Part model, mm, in its own coordinate system. A direction names the side the tool comes from. Coordinates: 2 decimals unless noted, no trailing zeros. Write each loop counter-clockwise with the first axis right and the second up, starting at its lowest first coordinate (ties: lowest second). Pieces come first, ordered by that corner, then holes. Notation, with made-up numbers: (-39.5, -27) - (14.5, -27) arc R33 cw to (14.5, 10) - close; hole circle Ø1 at (0, 43.25). An arc over 180 degrees is marked (long way). Write each question's results on one line, items separated by ' | '.
from build123d import *

# Parameters (mm, degrees)
SKETCH1_R           = 67.8
BOSS_EXTRUDE1_DEPTH = 20
SKETCH1_3_R         = 67.8
SKETCH1_3_R_2       = 50
BOSS_EXTRUDE2_DEPTH = 10


with BuildPart() as part:
    # Sketch1 → Boss-Extrude1 (new body)
    with BuildSketch(Plane(origin=(0, 0, 0), x_dir=(1, 0, 0), z_dir=(0, 1, 0))):
        with BuildLine():
            Line((242.754590009, 10), (260.147485469, 10))
            ThreePointArc((260.147485469, 10), (233.604843606, 39.180755583), (194.644031062, 33.009579084))
            ThreePointArc((194.644031062, 33.009579084), (161.546937037, 24.693656308), (132.733534149, 42.979170204))
            ThreePointArc((132.733534149, 42.979170204), (79.728157262, 75.530448258), (20.130518149, 57.718174568))
            ThreePointArc((20.130518149, 57.718174568), (-21.958648504, 36.745511037), (-68.95457192, 38.398915813))
            ThreePointArc((-68.95457192, 38.398915813), (-99.933181208, 34.770010311), (-118.888121928, 10))
            Line((-118.888121928, 10), (-103.07116694, 10))
            ThreePointArc((-103.07116694, 10), (-55.158288466, 0), (-103.07116694, -10))
            Line((-103.07116694, -10), (-118.888121928, -10))
            ThreePointArc((-118.888121928, -10), (-98.946037038, -35.313177478), (-66.810190141, -37.707138198))
            ThreePointArc((-66.810190141, -37.707138198), (-22.089611981, -34.732295435), (17.640354454, -55.476199781))
            ThreePointArc((17.640354454, -55.476199781), (75.663213782, -75.951962021), (129.887825017, -46.872749853))
            ThreePointArc((129.887825017, -46.872749853), (161.497288251, -27.924259237), (197.646050954, -35.098547889))
            ThreePointArc((197.646050954, -35.098547889), (235.316798867, -38.536697893), (260.147485469, -10))
            Line((260.147485469, -10), (242.754590009, -10))
            ThreePointArc((242.754590009, -10), (194.841711534, 0), (242.754590009, 10))
        make_face()
        with Locations(Location((69.841711534, 0, 0), (0, 0, 270))):
            Circle(SKETCH1_R, mode=Mode.SUBTRACT)
    extrude(amount=BOSS_EXTRUDE1_DEPTH)

    # Sketch1_3 → Boss-Extrude2 (add)
    with BuildSketch(Plane(origin=(0, 0, 0), x_dir=(1, 0, 0), z_dir=(0, 1, 0))):
        with Locations(Location((69.841711534, 0, 0), (0, 0, 270))):
            Circle(SKETCH1_3_R)
        with Locations(Location((69.841711534, 0, 0), (0, 0, 270))):
            Circle(SKETCH1_3_R_2, mode=Mode.SUBTRACT)
    extrude(amount=BOSS_EXTRUDE2_DEPTH)


solid = part.part
(1) Saw through at B-B on x = 88. Write the cut outline in (y, z).
Return value:
outline: (0, -73.98) - (20, -73.98) - (20, -65.32) - (10, -65.32) - (10, -46.59) - (0, -46.59) - close; (0, 46.59) - (10, 46.59) - (10, 65.32) - (20, 65.32) - (20, 73.98) - (0, 73.98) - close
(2) Saw through at A-A on z = 0. Write the cut outline in (x, y).
Return value:
outline: (-55.16, 0) - (19.84, 0) - (19.84, 10) - (2.04, 10) - (2.04, 20) - (-55.16, 20) - close; (119.84, 0) - (194.84, 0) - (194.84, 20) - (137.64, 20) - (137.64, 10) - (119.84, 10) - close
(3) 3-axis set-ups, long thin cutter, end or side, ignore diameter. For faces 1 (the flat face through (73, 0, -52)), 2 (the flat face through (19.9, 10, -5.3)), 3 (the flat face through (251, 10, -10)), 4 (the flat face through (-111, 10, -10)): which of +Z, -Z, +X, -X, +Y, -Y reach the whole face in a straight line?
Return value:
face 1: +Z, -Z, +X, -X, -Y | face 2: +Y | face 3: +X, +Y, -Y | face 4: -X, +Y, -Y
(4) Saw through at D-D on x = 220. Write the cut outline in (y, z).
Return value:
outline: (0, -41.53) - (20, -41.53) - (20, -25) - (0, -25) - close; (0, 25) - (20, 25) - (20, 41.53) - (0, 41.53) - close
(5) Flat gauge pins, fed straight in: P1, Ø1.5, axis at y = 9.5, z = 15, coming from the -X side; P2, Ø5, axis at x = -27.5, y = 5, coming from the +Z side; P3, Ø12, axis at x = 106, y = 3, coming from the -Z side. Where does each tip first touch, or does it go through?
Return value:
P1: stops at x = -117.53 | P2: stops at z = 34.17 | P3: stops at z = -69.95
(6) Saw through at C-C on y = 16.75. Write the cut outline in (x, z), then the cut area to 3 significant figures.
Return value:
outline: (-118.89, -10) arc R40 ccw to (-68.95, -38.4) arc R95.51 cw to (20.13, -57.72) arc R76.17 ccw to (132.73, -42.98) arc R43.22 cw to (194.64, -33.01) arc R41.53 ccw to (260.15, -10) - (242.75, -10) arc R25 cw (long way) to (242.75, 10) - (260.15, 10) arc R41.53 ccw to (197.65, 35.1) arc R51.23 cw to (129.89, 46.87) arc R76.17 ccw to (17.64, 55.48) arc R82.88 cw to (-66.81, 37.71) arc R40 ccw to (-118.89, 10) - (-103.07, 10) arc R25 cw (long way) to (-103.07, -10) - close; hole circle Ø135.6 at (69.84, 0) | area: 15,100 mm^2
(7) Two-plate mould, pull along Z, no slides. Class faces 5 (the cylindrical face through (-99.355, 9.86, 35.093)), 6 (the cylindrical face through (-99.54, 9.86, -34.99)), 7 (the flat face through (252, 10, 10)): released by +Z, released by -Z, zero draft, split by the parting line, or undercut.
Return value:
face 5: released by +Z | face 6: released by -Z | face 7: undercut
(8) Wall check: line 1 (X direction, y = 13.75, z = 0); line 2 (X direction, y = 5, z = 0); line 3 (Z direction, x = -94, y = 8.75). Give the ranges that are in metal, low to high. Write a range as from..to.
Return value:
line 1: x = -55.16..2.04, 137.64..194.84 | line 2: x = -55.16..19.84, 119.84..194.84 | line 3: z = -37.53..-20.82, 20.82..37.53
